For this review, take the finished solid that the model builds, in its own axes (mm). A direction names the side the tool comes from. Coordinates: 2 decimals unless noted, no trailing zeros. Loops run counter-clockwise (first coordinate to the right, second up) from the corner with the lowest first, then second, coordinate; pieces in that order, holes last. Notation, with made-up numbers: (41, 10.25) -> (86, 10.25) arc R29 cw to (86, 31.25) -> close; hole circle Ø3 at (25, 11). An arc over 180 degrees is marked (long way). Use a Markdown table: item, result.
Autodesk Fusion 360 part; units mm, degrees
sketch "Sketch1" plane through (0, 0, 0) normal (0, 0, 1) x (1, 0, 0)
  line L0 (-22.5, 22.5) -> (-22.5, -22.5)
  line L1 (-22.5, -22.5) -> (22.5, -22.5)
  line L2 (22.5, 16.9645) -> (22.5, 22.5)
  line L3 (-20, 20) -> (-20, 10.5061)
  line L4 (20, 20) -> (18.5858, 20)
  line L5 (-20, 20) -> (-22.5, 22.5)
  line L6 (-2.9289, 3.435) -> (15.5503, 21.9142)
  line L7 (22.5, 22.5) -> (16.9645, 22.5)
  line L8 (10.5061, -20) -> (20, -20)
  line L9 (20, -20) -> (22.5, -22.5)
  line L10 (3.435, -2.9289) -> (21.9142, 15.5503)
  line L11 (20, 18.5858) -> (20, 20)
  arc A0 (3.435, -2.9289) -> (10.5061, -20) centre (10.5061, -10) ccw
  arc A1 (-20, 10.5061) -> (-2.9289, 3.435) centre (-10, 10.5061) ccw
  line L12 (-18.5858, -20) -> (-20, -20)
  line L13 (-20, -18.5858) -> (-20, -20)
  line L14 (-18.5858, -20) -> (20, 18.5858)
  line L15 (-20, -18.5858) -> (18.5858, 20)
  arc A2 (21.9142, 15.5503) -> (22.5, 16.9645) centre (20.5, 16.9645) ccw
  arc A3 (16.9645, 22.5) -> (15.5503, 21.9142) centre (16.9645, 20.5) ccw
  line L16 (-20, 20) -> (-20, -18.5858)
  line L17 (20, -20) -> (-18.5858, -20)
  dimension "d3" = 45
  dimension "d4" = 45
  dimension "d5" = 10
  dimension "d6" = 2
extrude "Extrude1" add sketch "Sketch1" along normal blind 3 contours L0 L1 L3 L5 L8 L9 L12 L13 L16 L17 | L2 L4 L6 L7 L10 L11 A0 A1 L14 L15 A2 A3 L16 L17
extrude "Extrude2" add sketch "Sketch1" against normal blind 10 contours L0 L1 L3 L5 L8 L9 L12 L13 L16 L17
(1) For faces 4 (the face through (21, -21, -3)), 5 (the face through (16.189, 22.344, 1.479)), 6 (the face through (0.437, -0.977, 1.479)), list the 3-axis set-ups (+Z, -Z, +X, -X, +Y, -Y) from which the entire face can be reached by the end or side of a thin tool; tool diameter is ignored.
Found:
| item | result |
|---|---|
| face 4 | +Z, -Z, +X |
| face 5 | +Z, -Z, +Y |
| face 6 | +Z, -Z |
(2) Take a section at B-B on y = 14.5. Write out the cut boundary in (x, z).
Found:
| item | result |
|---|---|
| outline | (-22.5, -10) -> (-20, -10) -> (-20, 3) -> (-22.5, 3) -> close; (8.14, 0) -> (13.09, 0) -> (13.09, 3) -> (8.14, 3) -> close; (15.91, 0) -> (20.86, 0) -> (20.86, 3) -> (15.91, 3) -> close |
(3) Take a section at A-A on z = 1. Write out the cut boundary in (x, y) (1 decimal), plus the area to 3 significant figures.
Found:
| item | result |
|---|---|
| outline | (-22.5, -22.5) -> (22.5, -22.5) -> (20, -20) -> (10.5, -20) arc R10 cw to (3.4, -2.9) -> (21.9, 15.6) arc R2 ccw to (22.5, 17) -> (22.5, 22.5) -> (17, 22.5) arc R2 ccw to (15.6, 21.9) -> (-2.9, 3.4) arc R10 cw to (-20, 10.5) -> (-20, 20) -> (-22.5, 22.5) -> close; hole (-20, -20) -> (-18.6, -20) -> (20, 18.6) -> (20, 20) -> (18.6, 20) -> (-20, -18.6) -> close |
| area | 849 mm^2 |
(4) For pin 1 Ø8 at (x, y) = (-15, 16.5) entering from -Z; pin 2 Ø2 at (y, z) = (-6, -5) entering from +X; pin 3 Ø5 at (x, y) = (-5.5, -14) entering from -Z; pin 4 Ø6.5 at (x, z) = (0, -6.5) entering from +Y, all flat-tipped, find the tip position at first contact; note any pin that passes through.
Found:
| item | result |
|---|---|
| pin 1 | passes through |
| pin 2 | stops at x = -20 |
| pin 3 | stops at z = 0 |
| pin 4 | stops at y = -20 |
(5) Take a section at D-D on y = -7. Write out the cut boundary in (x, z).
Found:
| item | result |
|---|---|
| outline | (-22.5, -10) -> (-20, -10) -> (-20, 0) -> (-8.41, 0) -> (-8.41, 3) -> (-22.5, 3) -> close; (-5.59, 0) -> (0.97, 0) -> (0.97, 3) -> (-5.59, 3) -> close |
(6) Mouldability with a two-part tool opening along Y and no side actions: class faces 1 (the face through (22.352, 16.209, 1.479)), 2 (the face through (6.181, 12.545, 1.479)), 3 (the face through (22.5, 20, 1)) as pulls with the +Y half, pulls with the -Y half, needs draft (parallel to the pull), parting line crosses it, or undercut.
Found:
| item | result |
|---|---|
| face 1 | undercut |
| face 2 | pulls with the +Y half |
| face 3 | needs draft |
(7) Take a section at C-C on x = -18. Write out the cut boundary in (y, z).
Found:
| item | result |
|---|---|
| outline | (-22.5, -10) -> (-20, -10) -> (-20, 0) -> (-19.41, 0) -> (-19.41, 3) -> (-22.5, 3) -> close; (-16.59, 0) -> (4.51, 0) -> (4.51, 3) -> (-16.59, 3) -> close |
(8) For line 1 along X through (y, z) = (16, 2.25); line 2 along X through (y, z) = (11, 1); line 3 along Y through (x, z) = (-9, -7.75), list the stretches that pass through material, from the lowest coordinate up.
Found:
| item | result |
|---|---|
| line 1 | x = -22.5 to -20, 9.64 to 14.59, 17.41 to 22.25 |
| line 2 | x = -22.5 to -20, 4.64 to 9.59, 12.41 to 17.36 |
| line 3 | y = -22.5 to -20 |
